The drawing under review shows one solid part. Ordinate dimensions are in mm from its lowest x, y, z. Give positions to 0.01 mm unless a question says otherwise; leave off trailing zeros. Write each loop counter-clockwise with the first axis right and the second up, starting at its lowest first coordinate (ties: lowest second). Pieces come first, ordered by that corner, then holes. Notation, with made-up numbers: (88.5, 82.5) -> (135.5, 82.5) arc R35 ccw to (135.5, 121.5) -> close; hole circle Ø10 at (44.25, 18.5). An arc over 180 degrees is marked (long way). Use CSV: the item, a comma, the result in double quotes.
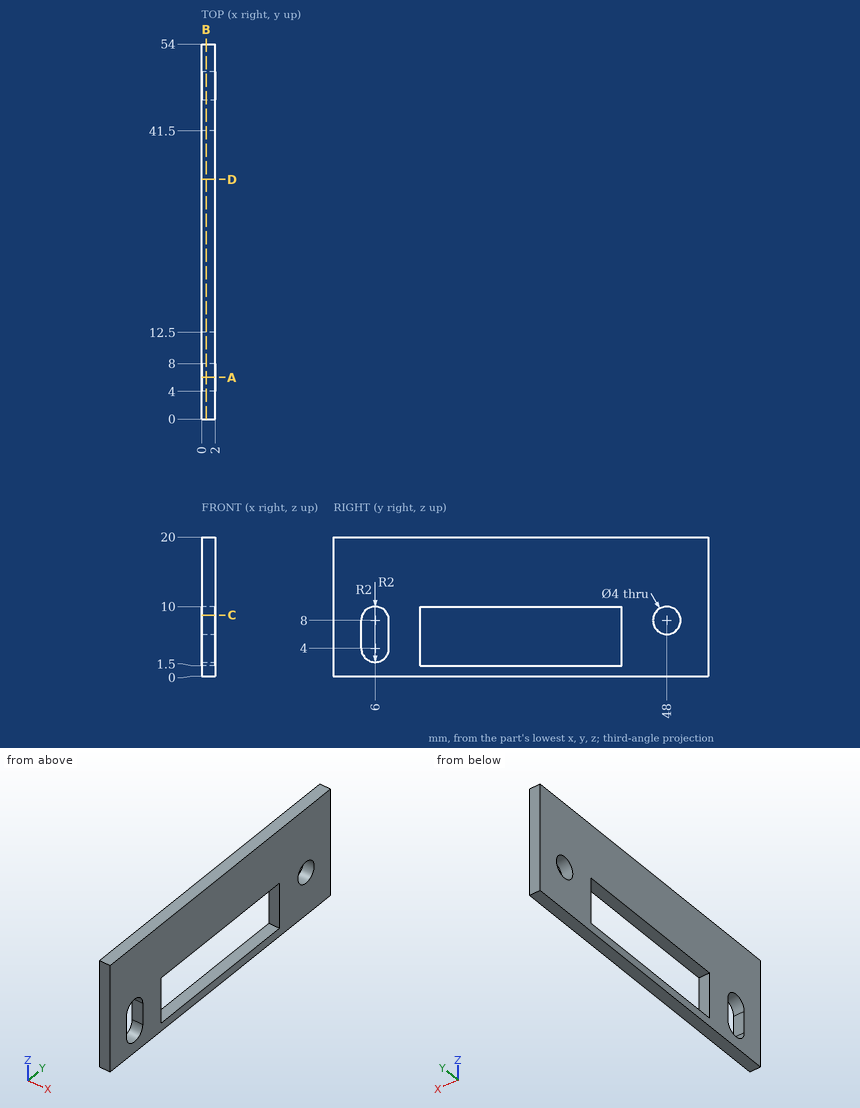
(1) For line 1 along Y through (x, z) = (1.3, 4.5); line 2 along Z through (x, y) = (0.45, 48); line 3 along Z through (x, y) = (1.45, 39.5), list the stretches that pass through material, from the lowest coordinate up. Write a range as [from, to].
Established:
line 1,"y = [0, 4], [8, 12.5], [41.5, 54]"
line 2,"z = [0, 6], [10, 20]"
line 3,"z = [0, 1.5], [10, 20]"
(2) Take a section at D-D (y = 34.5). Write out the cut boundary in (x, z).
Established:
outline,"(0, 0) -> (2, 0) -> (2, 1.5) -> (0, 1.5) -> close; (0, 10) -> (2, 10) -> (2, 20) -> (0, 20) -> close"
(3) Take a section at A-A (y = 6). Write out the cut boundary in (x, z), then the cut area to 3 significant figures.
Established:
outline,"(0, 0) -> (2, 0) -> (2, 2) -> (0, 2) -> close; (0, 10) -> (2, 10) -> (2, 20) -> (0, 20) -> close"
area,"24.0 mm2"
(4) Take a section at C-C (z = 8.75). Write out the cut boundary in (x, y).
Established:
outline,"(0, 0) -> (2, 0) -> (2, 4.15) -> (0, 4.15) -> close; (0, 7.85) -> (2, 7.85) -> (2, 12.5) -> (0, 12.5) -> close; (0, 41.5) -> (2, 41.5) -> (2, 46.15) -> (0, 46.15) -> close; (0, 49.85) -> (2, 49.85) -> (2, 54) -> (0, 54) -> close"
(5) Clearance check with a flat-ended pin moving along its axis: pin 1 (2.5 mm diameter, centred on y = 48, z = 8, fed in from -X). State where the tip first meets the part, or that it passes through.
Established:
pin 1,"passes through"
(6) Take a section at B-B (x = 0.65). Write out the cut boundary in (y, z).
Established:
outline,"(0, 0) -> (54, 0) -> (54, 20) -> (0, 20) -> close; hole (4, 4) arc R2 ccw to (8, 4) -> (8, 8) arc R2 ccw to (4, 8) -> close; hole (12.5, 1.5) -> (41.5, 1.5) -> (41.5, 10) -> (12.5, 10) -> close; hole circle Ø4 at (48, 8)"
